The listing builds one solid part. Answer for the finished solid, in the listing's coordinates (mm). A direction names the side the tool comes from. Give positions to 0.01 mm unless a question says otherwise; leave off trailing zeros. Order: outer loops, then holes, each group sorted by start corner. A loop starts at its lowest first (then second) coordinate and runs counter-clockwise, first axis right, second up. Notation, with made-up numbers: (47.5, -16.5) - (93.5, -16.5) arc R22 ccw to (93.5, -4.5) - close; hole circle Ø9 at (-33.5, 16). An arc over 180 degrees is marked (long way). Use a Markdown table: item, result. Add a question column.
1) Straight lines are drawn through the part: line 1 (Y direction, x = 84.5, z = 9.75) (3 decimals); line 2 (X direction, y = 16.5, z = 1.75); line 3 (X direction, y = 18.5, z = 2.75). For each, find the intervals that lie inside material, in ascending order.
2) Find section A-A, the plane x = -76.2. Determine the outline of the cut face in (y, z) (3 decimals).
3) Find section B-B, the plane x = 57.5. Determine the outline of the cut face in (y, z) (3 decimals), plus the area to 3 significant figures.
4) The mould has two halves that part along X. Classify faces 4 (the face through (1, 13, 3.175)), 5 (the face through (-37.22, 1.57, 10.03)), 6 (the face through (103.188, 14, 3)): released by +X, released by -X, zero draft, split by the parting line, or undercut.
5) For faces 1 (the face through (1, 13, 0)), 2 (the face through (1, 22.225, 11)), 3 (the face through (31.05, 23.83, 11.54)), determine the directions among +Z, -Z, +X, -X, +Y, -Y from which every point of the face is accessible in a straight line to the end or side of a thin tool.
6) Flat-ended cylindrical pins translate along their axes: pin 1 (10 mm diameter, centred on x = 76.2, y = 15.875, fed in from +Z) (3 decimals); pin 2 (4 mm diameter, centred on x = 34.925, z = 9.525, fed in from -Y). Find the tip coordinate at first contact, or state that the pin passes through.
from build123d import *

# Parameters (mm, degrees)
BOSS_EXTRUDE1_DEPTH = 103.1875
CUT_EXTRUDE2_REACH  = 109.962
SKETCH3_R           = 2.3495
CUT_EXTRUDE3_REACH  = 109.962
SKETCH4_R           = 4.36626
CUT_EXTRUDE4_REACH  = 109.962
SKETCH5_R           = 3.175


with BuildPart() as part:
    # Sketch1 → Boss-Extrude1 (new, symmetric)
    with BuildSketch(Plane(origin=(0, 0, 0), x_dir=(0, 0, -1), z_dir=(1, 0, 0))):
        Polygon((0, 25.4), (-19.05, 25.4), (-19.05, 22.225), (-3.175, 22.225), (-3.175, 3.175), (-19.05, 3.175), (-19.05, 0), (0, 0), align=None)
    extrude(amount=BOSS_EXTRUDE1_DEPTH, both=True)

    # Sketch3 → Cut-Extrude2 (cut, up to next)
    with BuildSketch(Plane.XZ, mode=Mode.PRIVATE) as cut_extrude2_sk1:
        with Locations(Location((34.925, 9.525, 0), (0, 0, 270))):
            Circle(SKETCH3_R)
    cut_extrude2_tool1 = extrude(cut_extrude2_sk1.sketch, amount=-CUT_EXTRUDE2_REACH, mode=Mode.PRIVATE) & part.part
    # Sketch3 → Cut-Extrude2 (cut, up to next)
    with BuildSketch(Plane.XZ, mode=Mode.PRIVATE) as cut_extrude2_sk2:
        with Locations(Location((-34.925, 9.525, 0), (0, 0, 270))):
            Circle(SKETCH3_R)
    cut_extrude2_tool2 = extrude(cut_extrude2_sk2.sketch, amount=-CUT_EXTRUDE2_REACH, mode=Mode.PRIVATE) & part.part
    add(cut_extrude2_tool1.solids().sort_by_distance((34.925, 0, 9.525))[0], mode=Mode.SUBTRACT)
    add(cut_extrude2_tool2.solids().sort_by_distance((-34.925, 0, 9.525))[0], mode=Mode.SUBTRACT)

    # Sketch4 → Cut-Extrude3 (cut, up to next)
    with BuildSketch(Plane(origin=(0, 25.4, 0), x_dir=(1, 0, 0), z_dir=(0, 1, 0)), mode=Mode.PRIVATE) as cut_extrude3_sk1:
        with Locations(Location((-34.925, -9.525, 0), (0, 0, 270))):
            Circle(SKETCH4_R)
    cut_extrude3_tool1 = extrude(cut_extrude3_sk1.sketch, amount=-CUT_EXTRUDE3_REACH, mode=Mode.PRIVATE) & part.part
    # Sketch4 → Cut-Extrude3 (cut, up to next)
    with BuildSketch(Plane(origin=(0, 25.4, 0), x_dir=(1, 0, 0), z_dir=(0, 1, 0)), mode=Mode.PRIVATE) as cut_extrude3_sk2:
        with Locations(Location((34.925, -9.525, 0), (0, 0, 270))):
            Circle(SKETCH4_R)
    cut_extrude3_tool2 = extrude(cut_extrude3_sk2.sketch, amount=-CUT_EXTRUDE3_REACH, mode=Mode.PRIVATE) & part.part
    add(cut_extrude3_tool1.solids().sort_by_distance((-34.925, 25.4, 9.525))[0], mode=Mode.SUBTRACT)
    add(cut_extrude3_tool2.solids().sort_by_distance((34.925, 25.4, 9.525))[0], mode=Mode.SUBTRACT)

    # Sketch5 → Cut-Extrude4 (cut, up to next)
    with BuildSketch(Plane(origin=(0, 0, 0), x_dir=(-1, 0, 0), z_dir=(0, 0, -1)), mode=Mode.PRIVATE) as cut_extrude4_sk1:
        with Locations((-76.2, 15.875)):
            Circle(SKETCH5_R)
    cut_extrude4_tool1 = extrude(cut_extrude4_sk1.sketch, amount=-CUT_EXTRUDE4_REACH, mode=Mode.PRIVATE) & part.part
    # Sketch5 → Cut-Extrude4 (cut, up to next)
    with BuildSketch(Plane(origin=(0, 0, 0), x_dir=(-1, 0, 0), z_dir=(0, 0, -1)), mode=Mode.PRIVATE) as cut_extrude4_sk2:
        with Locations((76.2, 15.875)):
            Circle(SKETCH5_R)
    cut_extrude4_tool2 = extrude(cut_extrude4_sk2.sketch, amount=-CUT_EXTRUDE4_REACH, mode=Mode.PRIVATE) & part.part
    add(cut_extrude4_tool1.solids().sort_by_distance((76.2, 15.875, 0))[0], mode=Mode.SUBTRACT)
    add(cut_extrude4_tool2.solids().sort_by_distance((-76.2, 15.875, 0))[0], mode=Mode.SUBTRACT)

    # Cut-Sweep1: sweep along a path in Sketch6
    with BuildLine(Plane(origin=(0, 25.4, 0), x_dir=(1, 0, 0), z_dir=(0, 1, 0))) as cut_sweep1_path:
        Line((-111.0615, 0.508), (-108.5215, 0.508))
        ThreePointArc((-108.5215, 0.508), (-103.492556572, -1.575056572), (-101.4095, -6.604))
        Line((-101.4095, -6.604), (-101.4095, -12.446))
        ThreePointArc((-101.4095, -12.446), (-103.492556572, -17.474943428), (-108.5215, -19.558))
        Line((-108.5215, -19.558), (-111.0615, -19.558))
    # Sketch7 → Cut-Sweep1 (sweep, cut)
    with BuildSketch(Plane(origin=(-111.0615, 25.4, -0.508), x_dir=(0, 0, -1), z_dir=(1, 0, 0))):
        Polygon((-4.572, -4.572), (-4.572, 0.508), (0.508, 0.508), align=None)
        Polygon((-4.572, -20.828), (-4.572, -25.908), (0.508, -25.908), align=None)
    cut_sweep1 = sweep(path=cut_sweep1_path.line, mode=Mode.SUBTRACT)

    # Mirror1: Cut-Sweep1 across plane
    add(cut_sweep1.mirror(Plane(origin=(0, 0, 0), x_dir=(0, 0, 1), z_dir=(1, 0, 0))), mode=Mode.SUBTRACT)


solid = part.part
The answers:
| question | item | result |
|---|---|---|
| 1 | line 1 | 0 to 3.175, 22.225 to 25.4 |
| 1 | line 2 | -103.19 to -79.31, -73.09 to 73.09, 79.31 to 103.19 |
| 1 | line 3 | -103.19 to -77.99, -74.41 to 74.41, 77.99 to 103.19 |
| 2 | outline | (0, 0) - (12.7, 0) - (12.7, 3.175) - (3.175, 3.175) - (3.175, 19.05) - (0, 19.05) - close; (19.05, 0) - (25.4, 0) - (25.4, 19.05) - (22.225, 19.05) - (22.225, 3.175) - (19.05, 3.175) - close |
| 3 | outline | (0, 0) - (25.4, 0) - (25.4, 19.05) - (22.225, 19.05) - (22.225, 3.175) - (3.175, 3.175) - (3.175, 19.05) - (0, 19.05) - close |
| 3 | area | 181 mm2 |
| 4 | face 4 | zero draft |
| 4 | face 5 | undercut |
| 4 | face 6 | released by +X |
| 5 | face 1 | -Z, +X, -X, +Y, -Y |
| 5 | face 2 | +Z, +X, -X |
| 5 | face 3 | +Y |
| 6 | pin 1 | z = 3.175 |
| 6 | pin 2 | through |
